Geometry: final body of the model. Coordinates: model frame, mm. Give positions to 0.01 mm unless a question says otherwise; leave off trailing zeros. Write each loop counter-clockwise with the first axis right and the second up, starting at its lowest first coordinate (ties: lowest second). Pieces come first, ordered by that corner, then holes. Notation, with made-up numbers: M -26,66 L 20,66 A32 ccw 20,96 Z; hole C -28.5,64.5 d3. An arc over 180 degrees is marked long. One line per question, with ' | ' between items.
Autodesk Inventor part; units mm, degrees
ref_plane "YZ Plane" through (0, 0, 0) normal (1, 0, 0) x (0, 1, 0)
ref_plane "XZ Plane" through (0, 0, 0) normal (0, 1, 0) x (-1, 0, 0)
ref_plane "XY Plane" through (0, 0, 0) normal (0, 0, 1) x (1, 0, 0)
sketch "Sketch1" plane through (0, 0, 0) normal (0, 1, 0) x (-1, 0, 0)
  line L0 (-2.1274, 0.9713) -> (2.9526, 0.9713)
  line L1 (2.9526, 0.9713) -> (2.9526, -1.5687)
  line L2 (2.9526, -1.5687) -> (-2.1274, -1.5687)
  line L3 (-2.1274, -1.5687) -> (-2.1274, 0.9713)
  point P0 (0, 0)
  dimension "d0" = 5.08
  dimension "d1" = 2.54
extrude "Extrusion1" add sketch "Sketch1" along normal blind 6.1
ref_plane "Work Plane1" through (1.4924, 0, 0.9713) normal (1, 0, 0) x (0, 0, -1)
sketch "Sketch2" plane through (1.4924, 0, 0.9713) normal (1, 0, 0) x (0, 0, -1)
  line L0 (3.24, 0) -> (-0.7, 0)
  line L1 (-0.7, 0) -> (-0.7, 0.48)
  line L2 (-0.7, 0.48) -> (3.24, 0.48)
  line L3 (3.24, 0.48) -> (3.24, 0)
  line L4 (0, 0) -> (0, 6.1)
  point P0 (0.9713, 0)
  dimension "d5" = 3.94
  dimension "d6" = 0.7
  dimension "d7" = 0.48
extrude "Extrusion2" add sketch "Sketch2" along normal mid plane 0.48
pattern_linear "Rectangular Pattern1" count 4 spacing 1.27 along (-1, 0, 0) of "Extrusion2"
sketch "Sketch3" plane through (0, 6.1, 0) normal (0, 1, 0) x (1, 0, 0)
  line L0 (2.1274, 1.5687) -> (-2.9526, 1.5687)
  line L1 (-2.9526, 1.5687) -> (-2.9526, -0.9713)
  line L2 (-2.5676, 0.5487) -> (-2.0676, 0.5487)
  line L3 (-2.0676, 0.5487) -> (-2.0676, 0.0487)
  line L4 (-2.0676, 0.0487) -> (-2.5676, 0.0487)
  line L5 (-2.5676, 0.0487) -> (-2.5676, 0.5487)
  point P0 (0, 0)
  dimension "d13" = 0.5
  dimension "d14" = 0.5
  dimension "d15" = 0.385
  dimension "d16" = 1.02
extrude "Extrusion3" cut sketch "Sketch3" against normal through all
pattern_linear "Rectangular Pattern2" count 4 spacing 1.27 along (1, 0, 0) of "Extrusion3"
properties part number "Recepticle_127"
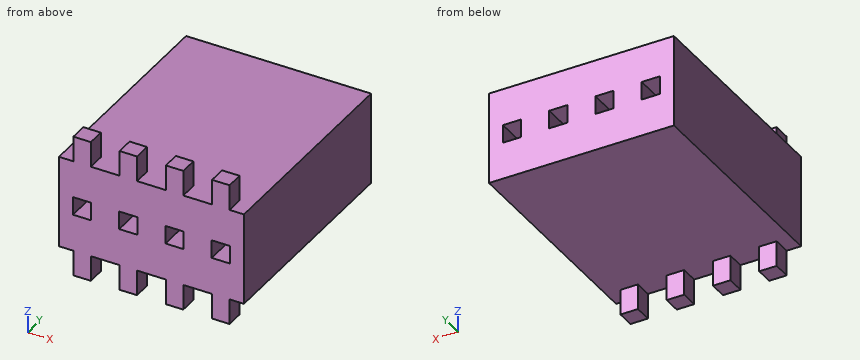
(1) Material intervals for L1, parallel to X at y = 1.25, z = -0.3; L2, parallel to Z at x = 1.65, y = 3.25; L3, parallel to Z at x = 0.9, y = 4.75, sorted ascending. Write a range as [from, to].
Working result:
L1: x = [-2.95, -2.57], [-2.07, -1.3], [-0.8, -0.03], [0.47, 1.24], [1.74, 2.13] | L2: z = [-1.57, -0.55], [-0.05, 0.97] | L3: z = [-1.57, 0.97]
(2) First-contact query: P1, Ø2.5, axis at x = -0.5, y = 3.5, coming from the +Z side; P2, Ø0.5, axis at x = 0.5, z = 1.5, coming from the +Y side. Flat tips, straight axial feed; report the tip coordinate or a pass-through.
Working result:
P1: stops at z = 0.97 | P2: stops at y = 0.48
(3) Cut plane D-D, the plane y = 4.5. Return loops of the section in (x, z), then the cut area to 3 significant figures.
Working result:
outline: M -2.95,-1.57 L 2.13,-1.57 L 2.13,0.97 L -2.95,0.97 Z; hole M -2.57,-0.55 L -2.07,-0.55 L -2.07,-0.05 L -2.57,-0.05 Z; hole M -1.3,-0.55 L -0.8,-0.55 L -0.8,-0.05 L -1.3,-0.05 Z; hole M -0.03,-0.55 L 0.47,-0.55 L 0.47,-0.05 L -0.03,-0.05 Z; hole M 1.24,-0.55 L 1.74,-0.55 L 1.74,-0.05 L 1.24,-0.05 Z | area: 11.9 mm^2
(4) Cut plane C-C, the plane z = -0.15. Return loops of the section in (x, y), then the cut area to 3 significant figures.
Working result:
outline: M -2.95,0 L -2.57,0 L -2.57,6.1 L -2.95,6.1 Z; M -2.07,0 L -1.3,0 L -1.3,6.1 L -2.07,6.1 Z; M -0.8,0 L -0.03,0 L -0.03,6.1 L -0.8,6.1 Z; M 0.47,0 L 1.24,0 L 1.24,6.1 L 0.47,6.1 Z; M 1.74,0 L 2.13,0 L 2.13,6.1 L 1.74,6.1 Z | area: 18.8 mm^2
(5) Cut plane A-A, the plane z = -1.65. Return loops of the section in (x, y), then the cut area to 3 significant figures.
Working result:
outline: M -2.56,0 L -2.08,0 L -2.08,0.48 L -2.56,0.48 Z; M -1.29,0 L -0.81,0 L -0.81,0.48 L -1.29,0.48 Z; M -0.02,0 L 0.46,0 L 0.46,0.48 L -0.02,0.48 Z; M 1.25,0 L 1.73,0 L 1.73,0.48 L 1.25,0.48 Z | area: 0.922 mm^2
(6) Cut plane B-B, the plane x = 0.1. Return loops of the section in (y, z).
Working result:
outline: M 0,-2.27 L 0.48,-2.27 L 0.48,-1.57 L 6.1,-1.57 L 6.1,-0.55 L 0,-0.55 Z; M 0,-0.05 L 6.1,-0.05 L 6.1,0.97 L 0.48,0.97 L 0.48,1.67 L 0,1.67 Z
